Build history of the part. All positions in model axes, mm. Round coordinates to 2 decimals unless told otherwise and drop trailing zeros. Order: outer loops, then holes, each group sorted by start corner. A loop starts at its lowest first (then second) coordinate and runs counter-clockwise, first axis right, second up. Notation, with made-up numbers: (29, 41.5) -> (87, 41.5) arc R20 cw to (87, 76.5) -> close; hole circle Ø4 at (46, -26.75). An arc over 180 degrees is marked (long way). Answer as a JSON object with one key per item and string values.
from build123d import *

# Parameters (mm, degrees)
BASENUTSKE_R  = 1.8
BASENUT_DEPTH = 3


with BuildPart() as part:
    # BaseNutSke → BaseNut (new body)
    with BuildSketch(Plane.XY):
        Polygon((2.95, 1.703183294), (2.95, -1.703183294), (0, -3.406366588), (-2.95, -1.703183294), (-2.95, 1.703183294), (0, 3.406366588), align=None)
        Circle(BASENUTSKE_R, mode=Mode.SUBTRACT)
    extrude(amount=-BASENUT_DEPTH)

    # Sketch3 → Double-Chamfer (revolve, cut)
    with BuildSketch(Plane(origin=(0, 0, 0), x_dir=(0, 0, -1), z_dir=(1, 0, 0))):
        Polygon((3, 2.75), (2.365, 3.406366588), (2.365, 16.106366588), (15.7, 16.106366588), (15.7, 2.75), align=None)
        Polygon((0.635, 16.106366588), (-12.7, 16.106366588), (-12.7, 2.75), (0, 2.75), (0.635, 3.406366588), align=None)
    revolve(axis=Axis((0, 0, 0), (0, 0, -1)), mode=Mode.SUBTRACT)

    # Sketch5 → EndChamfer (revolve, cut)
    with BuildSketch(Plane(origin=(0, 0, 0), x_dir=(0, 0, -1), z_dir=(1, 0, 0))):
        Polygon((2.9502, 2.5), (1.891136098, 0.9875), (3.001, 0.9875), (3.001, 2.5), align=None)
        Polygon((-0.002, 2.5), (0.0488, 2.5), (1.107863902, 0.9875), (-0.002, 0.9875), align=None)
    revolve(axis=Axis((0, 0, -25.037505729), (0, 0, -1)), mode=Mode.SUBTRACT)


solid = part.part
1) Pull direction X, two halves, no side cores. Call faces 1 (the face through (1.5, -2.54, -1.48)), 2 (the face through (-1.45, -2.57, -1.48)), 3 (the face through (0.831, -1.597, -1.486)): pulls with the +X half, pulls with the -X half, needs draft (parallel to the pull), parting line crosses it, or undercut.
Checked values:
{"face 1": "pulls with the +X half", "face 2": "pulls with the -X half", "face 3": "undercut"}
2) Cut at A-A, the plane z = -2.1. Give the cut face in (x, y).
Checked values:
{"outline": "(-2.95, -1.7) -> (0, -3.41) -> (2.95, -1.7) -> (2.95, 1.7) -> (0, 3.41) -> (-2.95, 1.7) -> close; hole circle Ø3.6 at (0, 0)"}
3) Cut at B-B, the plane y = 0. Give the cut face in (x, z), plus the area to 3 significant figures.
Checked values:
{"outline": "(-2.95, -2.81) -> (-2.75, -3) -> (-2.5, -3) -> (-2.5, -2.95) -> (-1.8, -2.46) -> (-1.8, -0.54) -> (-2.5, -0.05) -> (-2.5, 0) -> (-2.75, 0) -> (-2.95, -0.19) -> close; (1.8, -2.46) -> (2.5, -2.95) -> (2.5, -3) -> (2.75, -3) -> (2.95, -2.81) -> (2.95, -0.19) -> (2.75, 0) -> (2.5, 0) -> (2.5, -0.05) -> (1.8, -0.54) -> close", "area": "6.00 mm²"}
4) Probe L1, parallel to X at y = 0, z = -1; L2, parallel to Y at x = -0.9, z = -0.65; L3, parallel to Y at x = 0.35, z = -1.1. List the from-to ranges inside material, lowest first. Write a range as from..to.
Checked values:
{"L1": "x = -2.95..-1.8, 1.8..2.95", "L2": "y = -2.89..-1.56, 1.56..2.89", "L3": "y = -3.2..-1.77, 1.77..3.2"}
5) Flat gauge pin, fed straight in: pin 1 Ø1.5 at (x, y) = (0.5, -1.5) entering from -Z. Where does the tip first touch, or does it go through?
Checked values:
{"pin 1": "stops at z = -2.83"}
